```python
from build123d import *

# Parameters (mm, degrees)
BOSS_EXTRUDE1_DEPTH = 3.175
BOSS_EXTRUDE2_DEPTH = 3.175
LPATTERN1_COUNT     = 5
LPATTERN1_PITCH     = 109.22


with BuildPart() as part:
    # Sketch1 → Boss-Extrude1 (new body)
    with BuildSketch(Plane(origin=(0, 0, 0), x_dir=(1, 0, 0), z_dir=(0, 1, 0))):
        Polygon((0, 304.8), (0, 0), (508, 0), (508, 304.8), (53.593132378, 304.8), (7.268244995, 304.8), align=None)
    extrude(amount=BOSS_EXTRUDE1_DEPTH)

    # Sketch1<3> → Boss-Extrude2 (add)
    with BuildSketch(Plane(origin=(0, 0, 0), x_dir=(1, 0, 0), z_dir=(0, 1, 0))):
        with BuildLine():
            ThreePointArc((17.252367493, 309.650968343), (12.818348506, 306.076937756), (7.268244995, 304.8))
            Line((7.268244995, 304.8), (53.593132378, 304.8))
            ThreePointArc((53.593132378, 304.8), (48.043028868, 306.076937756), (43.609009881, 309.650968343))
            ThreePointArc((43.609009881, 309.650968343), (38.533476821, 318.209528266), (35.84709227, 327.790411412))
            ThreePointArc((35.84709227, 327.790411412), (36.197138958, 330.490776765), (37.891385065, 332.62245119))
            ThreePointArc((37.891385065, 332.62245119), (30.430688687, 355.6), (22.969992308, 332.62245119))
            ThreePointArc((22.969992308, 332.62245119), (24.664238415, 330.490776765), (25.014285104, 327.790411412))
            ThreePointArc((25.014285104, 327.790411412), (22.327900553, 318.209528266), (17.252367493, 309.650968343))
        make_face()
    boss_extrude2 = extrude(amount=BOSS_EXTRUDE2_DEPTH)

    # LPattern1: Boss-Extrude2 ×5
    with Locations(*[(i * LPATTERN1_PITCH, 0, 0) for i in range(1, LPATTERN1_COUNT)]):
        add(boss_extrude2)


solid = part.part
```
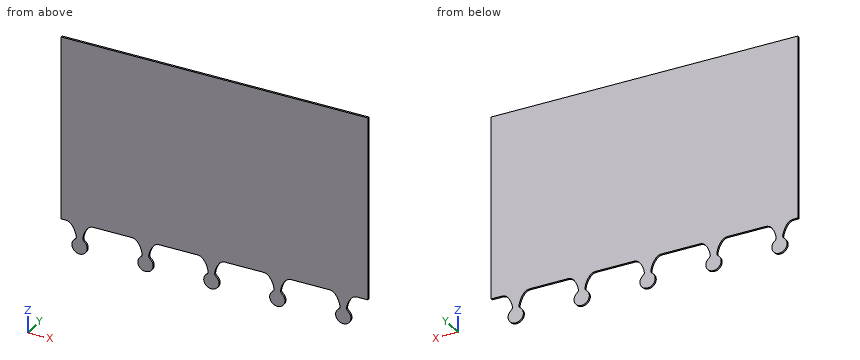
The listing builds one solid part. Answer for the finished solid, in the listing's coordinates (mm). Give positions to 0.01 mm unless a question says otherwise; leave off trailing zeros. Loops run counter-clockwise (first coordinate to the right, second up) from the corner with the lowest first, then second, coordinate; pieces in that order, holes last. Notation, with made-up numbers: (-1, 1) - (5, 1) arc R23 cw to (5, 30) - close; hole circle Ø4 at (9, 84). An arc over 180 degrees is marked (long way). Return JSON: item names as keys, results as strings. Group by question number.
1. Given pin 1 Ø1.6 at (x, y) = (500, 1.5) entering from -Z, flat-ended and moving along its own axis, determine where the tip first touches the part or whether it passes through.
2. Straight lines are drawn through the part: line 1 (Z direction, x = 290.5, y = 1.65); line 2 (Z direction, x = 347, y = 2.55); line 3 (Z direction, x = 29.5, y = 0.35). For each, find the intervals that lie inside material, in ascending order. Write a range as [from, to].
3. Find section A-A (z = -342.9). Write down the section's boundary in (x, y) (3 decimals).
4. Find section B-B (x = 319). Write down the section's boundary in (y, z) (3 decimals), then the cut area to 3 significant figures.
Verdict:
{
 "1": {"pin 1": "stops at z = -304.8"},
 "2": {"line 1": "z = [-304.8, 0]", "line 2": "z = [-349.09, -336.71], [-312.58, 0]", "line 3": "z = [-355.57, 0]"},
 "3": {"outline": "(17.731, 0) - (43.131, 0) - (43.131, 3.175) - (17.731, 3.175) - close; (126.951, 0) - (152.351, 0) - (152.351, 3.175) - (126.951, 3.175) - close; (236.171, 0) - (261.571, 0) - (261.571, 3.175) - (236.171, 3.175) - close; (345.391, 0) - (370.791, 0) - (370.791, 3.175) - (345.391, 3.175) - close; (454.611, 0) - (480.011, 0) - (480.011, 3.175) - (454.611, 3.175) - close"},
 "4": {"outline": "(0, -304.8) - (3.175, -304.8) - (3.175, 0) - (0, 0) - close", "area": "968 mm^2"}
}
